Autodesk Inventor part; units mm, degrees
ref_plane "YZ Plane" through (0, 0, 0) normal (1, 0, 0) x (0, 1, 0)
ref_plane "XZ Plane" through (0, 0, 0) normal (0, 1, 0) x (-1, 0, 0)
ref_plane "XY Plane" through (0, 0, 0) normal (0, 0, 1) x (1, 0, 0)
sketch "Sketch1" plane through (0, 0, 0) normal (1, 0, 0) x (0, 1, 0)
  line L0 (0, 0) -> (12.7, 0)
  line L1 (12.7, 0) -> (12.7, -18.034)
  line L2 (12.7, -18.034) -> (0, -18.034)
  line L3 (0, -18.034) -> (0, 0)
  line L4 (-3.175, 0) -> (15.875, 0)
  line L5 (15.875, 0) -> (15.875, -18.034)
  line L6 (15.875, -18.034) -> (-3.175, -18.034)
  line L7 (-3.175, -18.034) -> (-3.175, 0)
  circle A0 centre (2.54, -15.875) radius 0.715
  circle A1 centre (2.548, -2.159) radius 0.715
  circle A2 centre (10.168, -2.159) radius 0.715
  circle A3 centre (10.16, -15.875) radius 0.715
  circle A4 centre (6.35, -9.906) radius 3.5719
  circle A5 centre (6.35, -4.826) radius 1.5875
  point P0 (6.35, 0)
  point P1 (6.765, -6.3583)
  point P2 (5.935, -6.3583)
  dimension "d0" = 12.7
  dimension "d1" = 18.034
  dimension "d2" = 19.05
  dimension "d3" = 3.175
  dimension "d5" = 1.43
  dimension "d9" = 13.716
  dimension "d10" = 7.62
  dimension "d11" = 7.62
  dimension "d12" = 13.716
  dimension "d13" = 2.54
  dimension "d20" = 7.1437
  dimension "d21" = 3.175
  dimension "d23" = 2.159
  dimension "d24" = 2.159
extrude "Extrusion1" add sketch "Sketch1" along normal blind 0.762 contours L0 L1 L2 L3
properties part number "Base Top"
The listing builds one solid part. Answer for the finished solid, in the listing's coordinates (mm). Give positions to 0.01 mm unless a question says otherwise; leave off trailing zeros. Order: outer loops, then holes, each group sorted by start corner. A loop starts at its lowest first (then second) coordinate and runs counter-clockwise, first axis right, second up.
Item 1: Given pin 1 Ø2.5 at (y, z) = (2.548, -2.159) entering from -X, flat-ended and moving along its own axis, determine where the tip first touches the part or whether it passes through.
From the geometry:
pin 1: stops at x = 0
Item 2: The part is cut by section A-A, the plane z = -8.5. Give the vertices of the cut face in (x, y), and give its area (3 significant figures).
From the geometry:
outline: (0, 0) - (0.76, 0) - (0.76, 3.07) - (0, 3.07) - close; (0, 9.63) - (0.76, 9.63) - (0.76, 12.7) - (0, 12.7) - close
area: 4.67 mm2
Item 3: The part is cut by section D-D, the plane x = 0.2. Count the separate pieces of the cut face and the enclosed holes in it, and give its area (3 significant figures).
From the geometry:
separate pieces: 1
enclosed holes: 5
area: 175 mm2
Item 4: For a pull along Z with two mould halves and no side action, classify faces 1 (the face through (0.376, 2.447, -16.584)), 2 (the face through (0, 9, -7)) as pulls with the +Z half, pulls with the -Z half, needs draft (parallel to the pull), parting line crosses it, or undercut.
From the geometry:
face 1: undercut
face 2: needs draft
Item 5: The part is cut by section C-C, the plane y = 10.16. Give the vertices of the cut face in (x, z), and give its area (3 significant figures).
From the geometry:
outline: (0, -18.03) - (0.76, -18.03) - (0.76, -16.59) - (0, -16.59) - close; (0, -15.16) - (0.76, -15.16) - (0.76, -2.87) - (0, -2.87) - close; (0, -1.44) - (0.76, -1.44) - (0.76, 0) - (0, 0) - close
area: 11.6 mm2
Item 6: Find the intervals of material crossed by probe 1 along Z at (x, y) = (0.3, 10.16); probe 2 along Z at (x, y) = (0.05, 10.5); probe 3 along Z at (x, y) = (0.2, 6.35), in increasing order.
From the geometry:
probe 1: z = -18.03 to -16.59, -15.16 to -2.87, -1.44 to 0
probe 2: z = -18.03 to -16.5, -15.25 to -2.79, -1.53 to 0
probe 3: z = -18.03 to -13.48, -3.24 to 0
Item 7: The part is cut by section B-B, the plane y = 6.35. Give the vertices of the cut face in (x, z).
From the geometry:
outline: (0, -18.03) - (0.76, -18.03) - (0.76, -13.48) - (0, -13.48) - close; (0, -3.24) - (0.76, -3.24) - (0.76, 0) - (0, 0) - close
